Autodesk Inventor part; units mm, degrees
ref_plane "Work Plane2" through (0, 0, 190.5) normal (0, 0, 1) x (1, 0, 0)
ref_plane "YZ Plane" through (0, 0, 0) normal (1, 0, 0) x (0, 1, 0)
ref_plane "XZ Plane" through (0, 0, 0) normal (0, 1, 0) x (-1, 0, 0)
ref_plane "Work Plane1" through (0, 0, 0) normal (0, 0, 1) x (1, 0, 0)
sketch "Sketch1" plane through (0, 0, 0) normal (0, 0, 1) x (1, 0, 0)
  arc A0 (-113.2188, 0) -> (-109.7581, 3.4607) centre (-113.2188, 3.4607) ccw
  line L0 (-109.7581, 17.1767) -> (-109.7581, 3.4607)
  arc A1 (-109.7581, 17.1767) -> (-114.8063, 22.225) centre (-114.8063, 17.1767) ccw
  line L1 (-115.8223, 22.225) -> (-114.8063, 22.225)
  arc A2 (-115.8223, 22.225) -> (-119.2831, 18.7642) centre (-115.8223, 18.7642) ccw
  line L2 (-119.2831, 16.4211) -> (-119.2831, 18.7642)
  arc A3 (-119.2831, 16.4211) -> (-116.6161, 16.4211) centre (-117.9496, 16.4211) ccw
  line L3 (-116.6161, 18.7642) -> (-116.6161, 16.4211)
  arc A4 (-115.8223, 19.558) -> (-116.6161, 18.7642) centre (-115.8223, 18.7642) ccw
  line L4 (-114.8063, 19.558) -> (-115.8223, 19.558)
  arc A5 (-112.4251, 17.1767) -> (-114.8063, 19.558) centre (-114.8063, 17.1767) ccw
  line L5 (-112.4251, 3.4607) -> (-112.4251, 17.1767)
  arc A6 (-113.2188, 2.667) -> (-112.4251, 3.4607) centre (-113.2188, 3.4607) ccw
  line L6 (-147.5723, 2.667) -> (-113.2188, 2.667)
  arc A7 (-148.3661, 3.4607) -> (-147.5723, 2.667) centre (-147.5723, 3.4607) ccw
  line L7 (-148.3661, 17.1767) -> (-148.3661, 3.4607)
  arc A8 (-145.9848, 19.558) -> (-148.3661, 17.1767) centre (-145.9848, 17.1767) ccw
  line L8 (-144.9688, 19.558) -> (-145.9848, 19.558)
  arc A9 (-144.1751, 18.7642) -> (-144.9688, 19.558) centre (-144.9688, 18.7642) ccw
  line L9 (-144.1751, 16.4211) -> (-144.1751, 18.7642)
  arc A10 (-144.1751, 16.4211) -> (-141.5081, 16.4211) centre (-142.8416, 16.4211) ccw
  line L10 (-141.5081, 18.7642) -> (-141.5081, 16.4211)
  arc A11 (-141.5081, 18.7642) -> (-144.9688, 22.225) centre (-144.9688, 18.7642) ccw
  line L11 (-145.9848, 22.225) -> (-144.9688, 22.225)
  arc A12 (-145.9848, 22.225) -> (-151.0331, 17.1767) centre (-145.9848, 17.1767) ccw
  line L12 (-151.0331, 3.4607) -> (-151.0331, 17.1767)
  arc A13 (-151.0331, 3.4607) -> (-147.5723, 0) centre (-147.5723, 3.4607) ccw
  line L13 (-113.2188, 0) -> (-147.5723, 0)
  point P0 (0, 0)
extrude "Extrusion1" add sketch "Sketch1" along normal blind 381
ref_plane "Work Plane2" through (0, 0, 190.5) normal (0, 0, 1) x (1, 0, 0)
sketch "Sketch2" plane through (-147.5723, 0, 0) normal (0, -1, 0) x (1, 0, 0)
  line L0 (34.3535, 0) -> (0, 0) construction
  line L1 (17.1767, 0) -> (17.1767, 381) construction
  line L2 (0, 381) -> (34.3535, 381) construction
  line L3 (17.1767, 382.5875) -> (17.1767, 354.0125) construction
  line L4 (24.3205, 375.4438) -> (24.3205, 361.1562)
  line L5 (10.033, 361.1562) -> (10.033, 375.4438)
  arc A0 (24.3205, 375.4438) -> (10.033, 375.4438) centre (17.1767, 375.4438) ccw
  arc A1 (10.033, 361.1562) -> (24.3205, 361.1562) centre (17.1767, 361.1562) ccw
  point P0 (147.5723, 0)
  point P1 (17.1767, 368.3)
  dimension "d6" = 14.2875
  dimension "d7" = 28.575
  dimension "d15" = 1.5875
extrude "Extrusion2" cut sketch "Sketch2" against normal blind 25.4
pattern_linear "Rectangular Pattern1" count 8 spacing 50.8 along (0, 0, -1) of "Extrusion2"
properties part number "Horizontal-Unistrut-Tower-Connector-15 w holes"
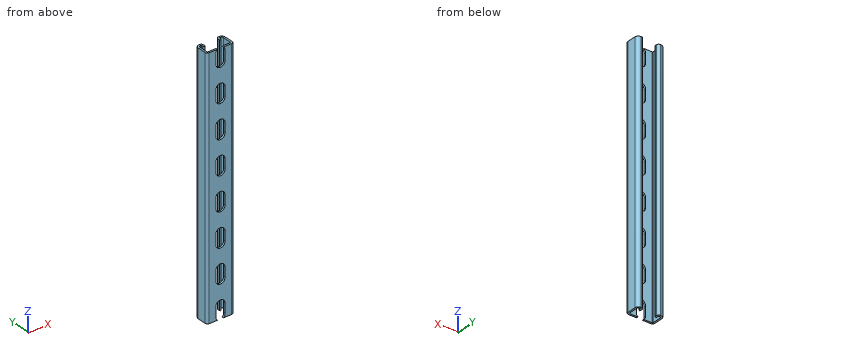
Verification items for the finished model (mm, model axes). Give positions to 0.01 mm unless a question says otherwise; leave off trailing zeros. Write each loop counter-clockwise with the first axis right and the second up, starting at its lowest first coordinate (ties: lowest second). Pieces come first, ordered by that corner, then holes. Notation, with made-up numbers: M 6.25,-33 L 46.25,-33 A17 ccw 46.25,-2 Z; hole C 85,-4.5 d9. An arc over 180 degrees is marked long. Use CSV: the item, a comma, the result in double quotes.
1) Cross-section at B-B (z = 239.5). Enter the section's corners in (x, y) (1 decimal), plus the area to 3 significant figures.
Final values:
outline,"M -151,3.5 A3.5 ccw -147.6,0 L -113.2,0 A3.5 ccw -109.8,3.5 L -109.8,17.2 A5 ccw -114.8,22.2 L -115.8,22.2 A3.5 ccw -119.3,18.8 L -119.3,16.4 A1.3 ccw -116.6,16.4 L -116.6,18.8 A0.8 cw -115.8,19.6 L -114.8,19.6 A2.4 cw -112.4,17.2 L -112.4,3.5 A0.8 cw -113.2,2.7 L -147.6,2.7 A0.8 cw -148.4,3.5 L -148.4,17.2 A2.4 cw -146,19.6 L -145,19.6 A0.8 cw -144.2,18.8 L -144.2,16.4 A1.3 ccw -141.5,16.4 L -141.5,18.8 A3.5 ccw -145,22.2 L -146,22.2 A5 ccw -151,17.2 Z"
area,"255 mm²"
2) Go/stop test with flat-tipped pins: pin 1 Ø3 at (x, z) = (-135, 210.5) entering from +Y; pin 2 Ø1.3 at (y, z) = (1.5, 217) entering from -X; pin 3 Ø5 at (x, z) = (-124.5, 114.5) entering from +Y; pin 4 Ø2 at (y, z) = (1.5, 371.5) entering from +X. Record where each tip stops, or that it passes through.
Final values:
pin 1,"through"
pin 2,"x = -150.78"
pin 3,"y = 2.67"
pin 4,"x = -109.89"
3) Material ranges on line 1 along X through (y, z) = (5.5, 351.5); line 2 along X through (y, z) = (16, 43); line 3 along Y through (x, z) = (-137, 249), recorded low to high.
Final values:
line 1,"-151.03 to -148.37, -112.43 to -109.76"
line 2,"-151.03 to -148.37, -144.11 to -141.58, -119.21 to -116.68, -112.43 to -109.76"
line 3,"0 to 2.67"
4) Cross-section at A-A (y = 7). Enter the section's corners in (x, z).
Final values:
outline,"M -151.03,0 L -148.37,0 L -148.37,381 L -151.03,381 Z; M -112.43,0 L -109.76,0 L -109.76,381 L -112.43,381 Z"
